Model file for the job. Use its own axes, mm. A direction names the side the tool comes from. Coordinates: 2 decimals unless noted, no trailing zeros. Order: outer loops, then holes, each group sorted by start corner. A loop starts at its lowest first (then second) coordinate and runs counter-clockwise, first axis right, second up. Notation, with made-up numbers: M -3.5,-10.5 L 2.5,-10.5 A32 cw 2.5,20.5 Z; hole C 49,40.5 d3. An arc over 180 degrees is marked long. Return JSON: item names as keys, results as strings.
```python
from build123d import *

# Parameters (mm, degrees)
F1_DEPTH     = 40
F0_W         = 8
F0_H         = 8
F0_R         = 1.425
F2_DEPTH     = 1.6
F3_R         = 2
F5_R         = 2
F6_START     = 30
F0_W_2       = 4
F0_H_2       = 4
F0_R_2       = 0.9
F6_DEPTH     = 8
F7_T1_DEPTH  = 8
F7_T6_DEPTH  = 4
F7_S7_R      = 0.9
F7_T8_DEPTH  = 4
F7_T13_DEPTH = 9
F7_T17_DEPTH = 13
F7_T24_DEPTH = 9
F7_T28_DEPTH = 13
F7_T31_DEPTH = 18


# Not quite as in the source:
# - a fillet or chamfer that OpenCascade refuses, or shapes differently, is made with other operations: its cross-section is extruded or revolved along the edge and cut away or added


with BuildPart() as f1:
    # F0 (on Front) → F1 (new body)
    with BuildSketch(Plane.XZ):
        Polygon((-26.6, -4.1515841149), (-26.6, -14.65), (-18.6, -14.65), (18.6, -14.65), (26.6, -14.65), (26.6, -4.1515841149), (26.6, 3.8484158851), (26.6, 14.65), (18.6, 14.65), (-18.6, 14.65), (-26.6, 14.65), (-26.6, 3.8484158851), align=None)
        Polygon((25, -2), (25, -13.05), (-25, -13.05), (-25, 13.05), (25, 13.05), (25, 2), align=None, mode=Mode.SUBTRACT)
    extrude(amount=F1_DEPTH)

    # F0 (on Front) → F2 (join)
    with BuildSketch(Plane.XZ):
        Polygon((-26.6, -4.1515841149), (-26.6, -14.65), (-18.6, -14.65), (18.6, -14.65), (26.6, -14.65), (26.6, -4.1515841149), (26.6, 3.8484158851), (26.6, 14.65), (18.6, 14.65), (-18.6, 14.65), (-26.6, 14.65), (-26.6, 3.8484158851), align=None)
        Polygon((25, -2), (25, -13.05), (-25, -13.05), (-25, 13.05), (25, 13.05), (25, 2), align=None, mode=Mode.SUBTRACT)
        with Locations((-22.6, -18.65)):
            Rectangle(F0_W, F0_H)
        with Locations((-22.6, -18.65)):
            Circle(F0_R, mode=Mode.SUBTRACT)
        with Locations((-30.6, -0.1515841149)):
            Rectangle(F0_W, F0_H)
        with Locations((-30.6, -0.1515841149)):
            Circle(F0_R, mode=Mode.SUBTRACT)
        with Locations((22.6, -18.65)):
            Rectangle(F0_W, F0_H)
        with Locations((22.6, -18.65)):
            Circle(F0_R, mode=Mode.SUBTRACT)
        with Locations((-22.6, 18.65)):
            Rectangle(F0_W, F0_H)
        with Locations((-22.6, 18.65)):
            Circle(F0_R, mode=Mode.SUBTRACT)
        with Locations((30.6, -0.1515841149)):
            Rectangle(F0_W, F0_H)
        with Locations((30.6, -0.1515841149)):
            Circle(F0_R, mode=Mode.SUBTRACT)
        with Locations((22.6, 18.65)):
            Rectangle(F0_W, F0_H)
        with Locations((22.6, 18.65)):
            Circle(F0_R, mode=Mode.SUBTRACT)
    extrude(amount=F2_DEPTH)

    # F3
    f3_edges = [f1.edges().sort_by_distance(p)[0] for p in [
        (-26.6, -0.8, 22.65),
        (-18.6, -0.8, 22.65),
        (18.6, -0.8, 22.65),
        (26.6, -0.8, 22.65),
        (34.6, -0.8, 3.848416),
        (34.6, -0.8, -4.151584),
        (26.6, -0.8, -22.65),
        (18.6, -0.8, -22.65),
        (-34.6, -0.8, -4.151584),
        (-34.6, -0.8, 3.848416),
        (-26.6, -0.8, -22.65),
    ]]
    fillet(f3_edges, radius=F3_R)

    # F4: F1 across plane


with BuildPart() as f1_1:
    add(f1.part)
    add(f1.part.mirror(Plane.YZ))

    # F5
    f5_edges = [f1_1.edges().sort_by_distance(p)[0] for p in [
        (-18.6, -0.8, -22.65),
        (18.6, -0.8, -22.65),
    ]]
    fillet(f5_edges, radius=F5_R)

    # F0 (on Front) → F6 (join)
    with BuildSketch(Plane.XZ.offset(F6_START)):
        with Locations((23, 0)):
            Rectangle(F0_W_2, F0_H_2)
        with Locations((23, 0)):
            Circle(F0_R_2, mode=Mode.SUBTRACT)
    extrude(amount=F6_DEPTH)

    # F7: fillet of radius 2 on 5 edges, made by hand

    # F7_s2 → F7_t1 (join)
    with BuildSketch(Plane.XZ.offset(30)):
        with BuildLine():
            ThreePointArc((25, -4), (24.4142135624, -2.5857864376), (23, -2))
            Line((23, -2), (25, -2))
            Line((25, -2), (25, -4))
        make_face()
        with BuildLine():
            ThreePointArc((25, 4), (24.4142135624, 2.5857864376), (23, 2))
            Line((23, 2), (25, 2))
            Line((25, 2), (25, 4))
        make_face()
    extrude(amount=F7_T1_DEPTH)


with BuildPart() as f7_tool4:
    # F7_s5 → F7_t6 (new body)
    with BuildSketch(Plane.XY.offset(-2)):
        with BuildLine():
            ThreePointArc((25, -28), (24.4142135624, -29.4142135624), (23, -30))
            Line((23, -30), (25, -30))
            Line((25, -30), (25, -28))
        make_face()
    extrude(amount=F7_T6_DEPTH)

    # F7_s7 → F7_t8 (cut, symmetric)
    with BuildSketch(Plane.XZ.offset(29)):
        with Locations((23, 0)):
            Circle(F7_S7_R)
    extrude(amount=F7_T8_DEPTH, both=True, mode=Mode.SUBTRACT)


with BuildPart() as f1_2:
    add(f1_1.part)

    # F7_t3: union F7_tool4
    add(f7_tool4.part)


with BuildPart() as f7_tool11:
    # F7_s12 → F7_t13 (new body)
    with BuildSketch(Plane.XY.offset(-7)):
        with BuildLine():
            ThreePointArc((25, -28), (24.4142135624, -29.4142135624), (23, -30))
            Line((23, -30), (25, -30))
            Line((25, -30), (25, -28))
        make_face()
    extrude(amount=F7_T13_DEPTH)

    split(bisect_by=Plane.XY.offset(-2), keep=Keep.BOTTOM)


with BuildPart() as f7_tool15:
    # F7_s16 → F7_t17 (new body)
    with BuildSketch(Plane.XZ.offset(25)):
        with BuildLine():
            ThreePointArc((25, -4), (24.4142135624, -2.5857864376), (23, -2))
            Line((23, -2), (25, -2))
            Line((25, -2), (25, -4))
        make_face()
    extrude(amount=F7_T17_DEPTH)

    split(bisect_by=Plane.XZ.offset(30), keep=Keep.BOTTOM)


with BuildPart() as f7_tool11_1:
    add(f7_tool11.part)

    # F7_t19: intersect F7_tool15
    add(f7_tool15.part, mode=Mode.INTERSECT)


with BuildPart() as f1_3:
    add(f1_2.part)

    # F7_t9: union F7_tool11
    add(f7_tool11_1.part)


with BuildPart() as f7_tool22:
    # F7_s23 → F7_t24 (new body)
    with BuildSketch(Plane.XY.offset(-2)):
        with BuildLine():
            ThreePointArc((25, -28), (24.4142135624, -29.4142135624), (23, -30))
            Line((23, -30), (25, -30))
            Line((25, -30), (25, -28))
        make_face()
    extrude(amount=F7_T24_DEPTH)

    split(bisect_by=Plane.XY.offset(2), keep=Keep.TOP)


with BuildPart() as f7_tool26:
    # F7_s27 → F7_t28 (new body)
    with BuildSketch(Plane.XZ.offset(25)):
        with BuildLine():
            ThreePointArc((25, 4), (24.4142135624, 2.5857864376), (23, 2))
            Line((23, 2), (25, 2))
            Line((25, 2), (25, 4))
        make_face()
    extrude(amount=F7_T28_DEPTH)

    split(bisect_by=Plane.XZ.offset(30), keep=Keep.BOTTOM)


with BuildPart() as f7_tool22_1:
    add(f7_tool22.part)

    # F7_t30: intersect F7_tool26
    add(f7_tool26.part, mode=Mode.INTERSECT)


with BuildPart() as f1_4:
    add(f1_3.part)

    # F7_t20: union F7_tool22
    add(f7_tool22_1.part)

    # F7_s32 → F7_t31 (cut)
    with BuildSketch(Plane.XZ.offset(25)):
        with BuildLine():
            ThreePointArc((23, -2), (21.5857864376, -1.4142135624), (21, 0))
            Line((21, 0), (21, -2))
            Line((21, -2), (23, -2))
        make_face()
        with BuildLine():
            ThreePointArc((23, 2), (21.5857864376, 1.4142135624), (21, 0))
            Line((21, 0), (21, 2))
            Line((21, 2), (23, 2))
        make_face()
    extrude(amount=F7_T31_DEPTH, mode=Mode.SUBTRACT)

    # F8: F1 across plane


with BuildPart() as f1_5:
    add(f1_4.part)
    add(f1_4.part.mirror(Plane.YZ))


solid = f1_5.part
```
Item 1: Saw through at C-C (y = -24.5). Write the cut outline in (x, z), and give its area (3 significant figures).
Check result:
{"outline": "M -26.6,-14.65 L 26.6,-14.65 L 26.6,14.65 L -26.6,14.65 Z; hole M -25,-13.05 L 25,-13.05 L 25,13.05 L -25,13.05 Z", "area": "254 mm2"}
Item 2: Drop flat-ended pins along their axis: pin 1 Ø1.8 at (x, y) = (-29, -1) entering from +Z; pin 2 Ø2 at (x, y) = (-24.5, -22.5) entering from -Z; pin 3 Ø13 at (y, z) = (-10, 5) entering from -X; pin 4 Ø6.5 at (x, z) = (20.5, -17.5) entering from -Y. Give the stop position or say it passes through.
Check result:
{"pin 1": "stops at z = 3.85", "pin 2": "stops at z = -14.65", "pin 3": "stops at x = -26.6", "pin 4": "stops at y = -40"}
Item 3: Pull direction Z, two halves, no side cores. Call faces 1 (the flat face through (23, -1, -22.65)), 2 (the flat face through (26.6, -20, 0)), 3 (the flat face through (25, -20, 0)), 4 (the flat face through (0, -20, -13.05)): +Z half, -Z half, draft (parallel to the pull), parting line (faces both ways), or undercut.
Check result:
{"face 1": "-Z half", "face 2": "draft", "face 3": "undercut", "face 4": "undercut"}
Item 4: Saw through at A-A (z = -10). Write the cut outline in (x, y), and give its area (3 significant figures).
Check result:
{"outline": "M -26.6,-40 L -25,-40 L -25,0 L -26.6,0 Z; M 25,-40 L 26.6,-40 L 26.6,0 L 25,0 Z", "area": "128 mm2"}
Item 5: Wall check: line 1 (X direction, y = -33, z = 0); line 2 (Z direction, x = 23, y = -34.75); line 3 (Z direction, x = -6.5, y = -2). Give the ranges that are in metal, low to high.
Check result:
{"line 1": "x = -26.6 to -23.9, -22.1 to -21, 21 to 22.1, 23.9 to 26.6", "line 2": "z = -14.65 to -13.05, -2 to -0.9, 0.9 to 2, 13.05 to 14.65", "line 3": "z = -14.65 to -13.05, 13.05 to 14.65"}
Item 6: 3-axis set-ups, long thin cutter, end or side, ignore diameter. For faces 5 (the flat face through (18.6, -1, 18)), 6 (the cylindrical face through (-24.65, -29.13, -0.06)), 7 (the flat face through (-23, -1.6, 17)), 8 (the flat face through (23, -1.6, -17)), 9 (the flat face through (-30, -1, 3.848)): which of +Z, -Z, +X, -X, +Y, -Y reach the whole face in a straight line?
Check result:
{"face 5": "+Z, +Y, -Y", "face 6": "+Y", "face 7": "+Z, +X, -X, -Y", "face 8": "-Z, +X, -X, -Y", "face 9": "+Z, -X, +Y, -Y"}
Item 7: Saw through at B-B (x = 16). Write the cut outline in (y, z).
Check result:
{"outline": "M -40,-14.65 L 0,-14.65 L 0,-13.05 L -40,-13.05 Z; M -40,13.05 L 0,13.05 L 0,14.65 L -40,14.65 Z"}
